from build123d import *

# Parameters (mm, degrees)
BOSS_EXTRU_1_DEPTH      = 11
ESQUISSE2_R             = 2.75
BOSS_EXTRU_2_DEPTH      = 1.5
BOSS_EXTRU_3_START      = 1.5
ESQUISSE3_R             = 2.75
BOSS_EXTRU_3_DEPTH      = 1.5
ESQUISSE5_W             = 7.8
ESQUISSE5_H             = 40.529247283
ENL_V_MAT_EXTRU_1_DEPTH = 10.5
ESQUISSE6_W             = 7.8
ESQUISSE6_H             = 5
ENL_V_MAT_EXTRU_2_DEPTH = 8
ESQUISSE7_W             = 7.8
ESQUISSE7_H             = 34.280292999
ENL_V_MAT_EXTRU_3_DEPTH = 8


with BuildPart() as part:
    # Esquisse1 → Boss.-Extru.1 (new body)
    with BuildSketch(Plane.XY):
        with BuildLine():
            Line((4, 2.561737691), (4, 39.561737691))
            Line((4, 39.561737691), (2, 40.679247283))
            Line((2, 40.679247283), (-3.5, 7.127049143))
            Line((-3.5, 7.127049143), (-2, 6.193131027))
            Line((-2, 6.193131027), (-4, 2.561737691))
            ThreePointArc((-4, 2.561737691), (0, -4.75), (4, 2.561737691))
        make_face()
    extrude(amount=BOSS_EXTRU_1_DEPTH)

    # Esquisse2 → Boss.-Extru.2 (add)
    with BuildSketch(Plane.XY):
        Circle(ESQUISSE2_R)
    extrude(amount=-BOSS_EXTRU_2_DEPTH)

    # Esquisse3 → Boss.-Extru.3 (add)
    with BuildSketch(Plane.XY.offset(11).offset(BOSS_EXTRU_3_START)):
        Circle(ESQUISSE3_R)
    extrude(amount=-BOSS_EXTRU_3_DEPTH)

    # Esquisse5 → Enlèv. mat.-Extru.1 (cut)
    with BuildSketch(Plane(origin=(14, 0, 0), x_dir=(0, 0, -1), z_dir=(1, 0, 0))):
        with Locations((-5.5, 17.414623642)):
            Rectangle(ESQUISSE5_W, ESQUISSE5_H)
    extrude(amount=-ENL_V_MAT_EXTRU_1_DEPTH, mode=Mode.SUBTRACT)

    # Esquisse6 → Enlèv. mat.-Extru.2 (cut)
    with BuildSketch(Plane(origin=(4.607784726, -2.537750279, 0), x_dir=(0, 0, 1), z_dir=(-0.8759373234553582, 0.4824249220115637, 0))):
        with Locations((5.5, 1.836793332)):
            Rectangle(ESQUISSE6_W, ESQUISSE6_H)
    extrude(amount=ENL_V_MAT_EXTRU_2_DEPTH, mode=Mode.SUBTRACT)

    # Esquisse7 → Enlèv. mat.-Extru.3 (cut)
    with BuildSketch(Plane(origin=(5.322160432, -0.872428157, 0), x_dir=(0, 0, 1), z_dir=(-0.986829357047507, 0.16176470588235298, 0))):
        with Locations((5.5, 20.689899695)):
            Rectangle(ESQUISSE7_W, ESQUISSE7_H)
    extrude(amount=ENL_V_MAT_EXTRU_3_DEPTH, mode=Mode.SUBTRACT)


solid = part.part
Geometry: final body of the model. Coordinates: model frame, mm. A direction names the side the tool comes from. Give positions to 0.01 mm unless a question says otherwise; leave off trailing zeros. Write each loop counter-clockwise with the first axis right and the second up, starting at its lowest first coordinate (ties: lowest second). Pieces come first, ordered by that corner, then holes. Notation, with made-up numbers: (25.25, 63.5) - (72.25, 63.5) arc R26 ccw to (72.25, 86.5) - close; hole circle Ø3 at (-13, 39). An arc over 180 degrees is marked (long way). Return JSON: item names as keys, results as strings. Group by question number.
1) Line query: line 1 (Z direction, x = 3.5, y = 35); line 2 (Z direction, x = 2, y = 0.5); line 3 (Z direction, x = -3.25, y = 3.5). Output: solid intervals per line, ascending.
2) Set-up query: faces 5 (the flat face through (-2.76, 6.667, 5.423)), 6 (the cylindrical face through (-0.596, -2.685, 11.76)), 7 (the flat face through (2, 13, 9.4)), 8 (the cylindrical face through (-0.596, -2.685, -0.74)). Return all of +Z, -Z, +X, -X, +Y, -Y with unobstructed straight access to the full face (end or side cutting, diameter ignored); none if empty.
3) First-contact query: P1, Ø5, axis at x = -0.5, z = 1.5, coming from the -Y side; P2, Ø3, axis at x = 2.5, y = 8, coming from the -Z side; P3, Ø3, axis at x = 2.5, y = 15, coming from the +Z side; P4, Ø5, axis at x = -3.5, y = 27, coming from the -Z side. Flat tips, straight axial feed; report the tip coordinate or a pass-through.
4) Mould query, pull axis Y, two halves, no side actions, for faces 1 (the flat face through (0, 0, -1.5)), 2 (the flat face through (-1.87, 2.28, 5.45)), 3 (the flat face through (0.434, -0.996, 5.445)), 4 (the cylindrical face through (-2.301, -4.156, 5.423)). Classes: released by +Y, released by -Y, zero draft, split by the parting line, or undercut.
5) Section B-B on x = 0. Return the cut outline in (y, z), plus the area to 3 significant figures.
6) Section D-D on y = 0. Return the cut outline in (x, z).
7) Section C-C on y = 18.5. Return the cut outline in (x, z).
Filled in:
{
 "1": {"line 1": "z = 0 to 1.6, 9.4 to 11", "line 2": "z = -1.5 to 1.6, 9.4 to 12.5", "line 3": "z = 0 to 11"},
 "2": {"face 5": "+Z, -Z, -X", "face 6": "+Z", "face 7": "+X", "face 8": "-Z"},
 "3": {"P1": "stops at y = -4.75", "P2": "stops at z = 0", "P3": "stops at z = 11", "P4": "passes through"},
 "4": {"face 1": "zero draft", "face 2": "undercut", "face 3": "undercut", "face 4": "split by the parting line"},
 "5": {"outline": "(-4.75, 0) - (-2.75, 0) - (-2.75, -1.5) - (2.75, -1.5) - (2.75, 0) - (28.48, 0) - (28.48, 11) - (2.75, 11) - (2.75, 12.5) - (-2.75, 12.5) - (-2.75, 11) - (-4.75, 11) - close; hole (-0.76, 1.6) - (16.11, 1.6) - (16.11, 9.4) - (-0.76, 9.4) - close", "area": "250 mm^2"},
 "6": {"outline": "(-4.75, 0) - (-2.75, 0) - (-2.75, -1.5) - (2.75, -1.5) - (2.75, 0) - (4.75, 0) - (4.75, 1.6) - (-1.37, 1.6) - (-1.37, 9.4) - (4.75, 9.4) - (4.75, 11) - (2.75, 11) - (2.75, 12.5) - (-2.75, 12.5) - (-2.75, 11) - (-4.75, 11) - close"},
 "7": {"outline": "(-1.64, 0) - (4, 0) - (4, 1.6) - (0.39, 1.6) - (0.39, 9.4) - (4, 9.4) - (4, 11) - (-1.64, 11) - close"}
}
